from build123d import *

# Parameters (mm, degrees)
SKETCH_W        = 125
SKETCH_H        = 155
PAD_DEPTH       = 5
SKETCH001_R     = 2.5
POCKET_DEPTH    = 5.001
SKETCH002_W     = 16.5
SKETCH002_H     = 52
POCKET001_DEPTH = 5.001
SKETCH003_R     = 11.5
SKETCH003_R_2   = 2.5
POCKET002_DEPTH = 5.001
SKETCH004_R     = 2.5
POCKET003_DEPTH = 5.001
SKETCH005_R     = 2.5
POCKET004_DEPTH = 5.001


with BuildPart() as part:
    # Sketch → Pad (new body)
    with BuildSketch(Plane.XY):
        Rectangle(SKETCH_W, SKETCH_H)
    extrude(amount=PAD_DEPTH)

    # Sketch001 (on Face6 of Pad) → Pocket (cut, through all)
    with BuildSketch(Plane.XY.offset(5)):
        with Locations((-47.5, 62.5)):
            Circle(SKETCH001_R)
        with Locations((47.5, 62.5)):
            Circle(SKETCH001_R)
        with Locations((-47.5, -62.5)):
            Circle(SKETCH001_R)
        with Locations((47.5, -62.5)):
            Circle(SKETCH001_R)
    extrude(amount=-POCKET_DEPTH, mode=Mode.SUBTRACT)

    # Sketch002 (on Face5 of Pocket) → Pocket001 (cut, through all)
    with BuildSketch(Plane.XY.offset(5)):
        with Locations((12.7, -15.5)):
            Rectangle(SKETCH002_W, SKETCH002_H)
    extrude(amount=-POCKET001_DEPTH, mode=Mode.SUBTRACT)

    # Sketch003 (on Face5 of Pocket001) → Pocket002 (cut, through all)
    with BuildSketch(Plane.XY.offset(5)):
        with Locations((12.7, 47.5)):
            Circle(SKETCH003_R)
        with Locations((-2.8, 63)):
            Circle(SKETCH003_R_2)
        with Locations((28.2, 63)):
            Circle(SKETCH003_R_2)
        with Locations((28.2, 32)):
            Circle(SKETCH003_R_2)
        with Locations((-2.8, 32)):
            Circle(SKETCH003_R_2)
    extrude(amount=-POCKET002_DEPTH, mode=Mode.SUBTRACT)

    # Sketch004 (on Face5 of Pocket002) → Pocket003 (cut, through all)
    with BuildSketch(Plane.XY.offset(5)):
        with Locations((8.7, -45.5)):
            Circle(SKETCH004_R)
        with Locations((16.7, -45.5)):
            Circle(SKETCH004_R)
    extrude(amount=-POCKET003_DEPTH, mode=Mode.SUBTRACT)

    # Sketch005 (on Face5 of Pocket003) → Pocket004 (cut, through all)
    with BuildSketch(Plane.XY.offset(5)):
        with Locations((26.7, 20)):
            Circle(SKETCH005_R)
        with Locations((54.7, 20)):
            Circle(SKETCH005_R)
        with Locations((26.7, -25.5)):
            Circle(SKETCH005_R)
        with Locations((54.7, -25.5)):
            Circle(SKETCH005_R)
        with Locations((-1.3, 20)):
            Circle(SKETCH005_R)
        with Locations((-29.3, 20)):
            Circle(SKETCH005_R)
        with Locations((-29.3, -25.5)):
            Circle(SKETCH005_R)
        with Locations((-1.3, -25.5)):
            Circle(SKETCH005_R)
    extrude(amount=-POCKET004_DEPTH, mode=Mode.SUBTRACT)


solid = part.part
Design review of the part built by this model. Coordinates are the model's own, in mm. A direction names the side the tool comes from. Coordinates: 2 decimals unless noted, no trailing zeros. Order: outer loops, then holes, each group sorted by start corner. A loop starts at its lowest first (then second) coordinate and runs counter-clockwise, first axis right, second up. Notation, with made-up numbers: M 4.5,44 L 47.5,44 A6 cw 47.5,50 Z; hole C -24.5,52 d6. An arc over 180 degrees is marked long. Use a Markdown table: item, result.
(1) For P1, Ø6.5, axis at x = 16.7, y = -45.5, coming from the +Z side, flat-tipped, find the tip position at first contact; note if it passes through.
Worked answers:
| item | result |
|---|---|
| P1 | stops at z = 5 |
(2) Add section B-B (x = 54.7). Give the boundary of the cut face in (y, z).
Worked answers:
| item | result |
|---|---|
| outline | M -77.5,0 L -28,0 L -28,5 L -77.5,5 Z; M -23,0 L 17.5,0 L 17.5,5 L -23,5 Z; M 22.5,0 L 77.5,0 L 77.5,5 L 22.5,5 Z |
(3) Draft analysis for pull direction X (two halves, no side actions). For faces 3 (the cylindrical face through (24.86, 21.69, 2.54)), 4 (the flat face through (-62.5, -1, 2)), 5 (the flat face through (-1, 1, 5)), state which applies: released by +X, released by -X, zero draft, split by the parting line, or undercut.
Worked answers:
| item | result |
|---|---|
| face 3 | undercut |
| face 4 | released by -X |
| face 5 | zero draft |
(4) Wall thickness on probe 1 along X at (y, z) = (-1.5, 2.35); probe 2 along Y at (x, z) = (47.5, 2.9); probe 3 along Y at (x, z) = (18.5, 0.95): over which ranges is each line inside the solid? List them lowest first.
Worked answers:
| item | result |
|---|---|
| probe 1 | x = -62.5 to 4.45, 20.95 to 62.5 |
| probe 2 | y = -77.5 to -65, -60 to 60, 65 to 77.5 |
| probe 3 | y = -77.5 to -47.23, -43.77 to -41.5, 10.5 to 37.57, 57.43 to 77.5 |
(5) For faces 1 (the flat face through (-1, -77.5, 2)), 2 (the flat face through (20.95, -16, 3)), list the 3-axis set-ups (+Z, -Z, +X, -X, +Y, -Y) from which the entire face can be reached by the end or side of a thin tool; tool diameter is ignored.
Worked answers:
| item | result |
|---|---|
| face 1 | +Z, -Z, +X, -X, -Y |
| face 2 | +Z, -Z |
(6) Add section A-A (y = 20). Give the boundary of the cut face in (x, z).
Worked answers:
| item | result |
|---|---|
| outline | M -62.5,0 L -31.8,0 L -31.8,5 L -62.5,5 Z; M -26.8,0 L -3.8,0 L -3.8,5 L -26.8,5 Z; M 1.2,0 L 24.2,0 L 24.2,5 L 1.2,5 Z; M 29.2,0 L 52.2,0 L 52.2,5 L 29.2,5 Z; M 57.2,0 L 62.5,0 L 62.5,5 L 57.2,5 Z |
(7) Add section D-D (x = 16.7). Give the boundary of the cut face in (y, z).
Worked answers:
| item | result |
|---|---|
| outline | M -77.5,0 L -48,0 L -48,5 L -77.5,5 Z; M -43,0 L -41.5,0 L -41.5,5 L -43,5 Z; M 10.5,0 L 36.72,0 L 36.72,5 L 10.5,5 Z; M 58.28,0 L 77.5,0 L 77.5,5 L 58.28,5 Z |
(8) Add section C-C (y = -62.5). Give the boundary of the cut face in (x, z), then the cut area to 3 significant figures.
Worked answers:
| item | result |
|---|---|
| outline | M -62.5,0 L -50,0 L -50,5 L -62.5,5 Z; M -45,0 L 45,0 L 45,5 L -45,5 Z; M 50,0 L 62.5,0 L 62.5,5 L 50,5 Z |
| area | 575 mm2 |
